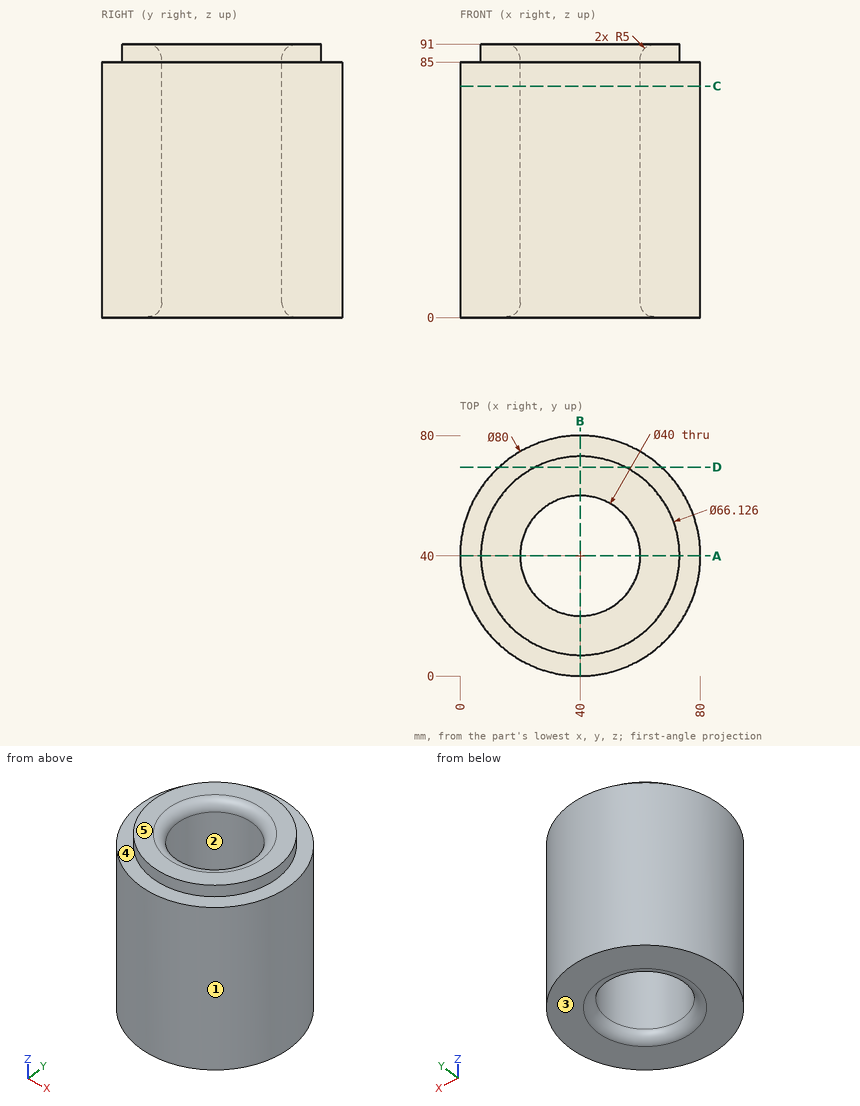
The figure shows three views and two pictorial views of one solid part (mm, origin at its lowest corner). Answer the questions. A direction names the side the tool comes from. Coordinates: 2 decimals unless noted, no trailing zeros. Loops run counter-clockwise (first coordinate to the right, second up) from the corner with the lowest first, then second, coordinate; pieces in that order, holes last.
1) Find section A-A on y = 40. Write down the section's boundary in (x, z), then the cut area to 3 significant figures.
2) Find the intervals of material crossed by L1, parallel to Y at x = 40, z = 63.5; L2, parallel to Z at x = 74.5, y = 60; L3, parallel to X at y = 54, z = 75.5, in increasing order.
3) Find section C-C on z = 77. Write down the section's boundary in (x, y), then the cut area to 3 significant figures.
4) Determine the mould class of the marked faces 1, 2 and 3 for opening direction Y: pulls with the +Y half, pulls with the -Y half, needs draft (parallel to the pull), parting line crosses it, or undercut.
5) Flat-ended cylindrical pins translate along their axes: pin 1 Ø12 at (y, z) = (58, 52.5) entering from -X; pin 2 Ø5 at (x, z) = (63.5, 35) entering from +Y; pin 3 Ø3 at (y, z) = (42.5, 21.5) entering from -X. Find the tip coordinate at first contact, or state that the pin passes through.
6) Find section D-D on y = 69.5. Write down the section's boundary in (x, z).
7) A tool of negligible diameter and unlimited length cuts with its end or side. For the marked faces 4 and 5, from which of +Z, -Z, +X, -X, +Y, -Y can it reach the whole face along a straight path? Write none if from no direction.
Values:
1. outline: (0, 0) - (15, 0) arc R5 ccw to (20, 5) - (20, 86) arc R5 ccw to (15, 91) - (6.94, 91) - (6.94, 85) - (0, 85) - close; (60, 5) arc R5 ccw to (65, 0) - (80, 0) - (80, 85) - (73.06, 85) - (73.06, 91) - (65, 91) arc R5 ccw to (60, 86) - close
1. area: 3,540 mm2
2. L1: y = 0 to 20, 60 to 80
2. L2: z = 0 to 85
2. L3: x = 2.53 to 25.72, 54.28 to 77.47
3. outline: circle Ø80 at (40, 40); hole circle Ø40 at (40, 40)
3. area: 3,770 mm2
4. face 1: parting line crosses it
4. face 2: undercut
4. face 3: needs draft
5. pin 1: stops at x = 1.84
5. pin 2: stops at y = 74.04
5. pin 3: stops at x = 0.01
6. outline: (12.99, 0) - (67.01, 0) - (67.01, 85) - (54.93, 85) - (54.93, 91) - (25.07, 91) - (25.07, 85) - (12.99, 85) - close
7. face 4: +Z
7. face 5: +Z, +X, -X, +Y, -Y
